The model under review builds one solid part; all positions refer to its coordinate system, in mm. A direction names the side the tool comes from. Round coordinates to 2 decimals unless told otherwise and drop trailing zeros. Order: outer loops, then holes, each group sorted by start corner. A loop starts at its lowest first (then second) coordinate and runs counter-clockwise, first axis right, second up. Notation, with made-up numbers: (-14, -34.5) - (6, -34.5) arc R5 ccw to (6, -28.5) - close; hole circle Ø9 at (29.25, -3.75). An arc over 180 degrees is marked (long way). One line per question, with ' | ' between items. Start each with the question number.
Item 1: Add section C-C on y = -4.25. State the section outline as (x, z) points.
Item 2: Draft analysis for pull direction Z (two halves, no side actions). For faces 3 (the face through (6.37, -0.94, 44.74)), 4 (the face through (4, -11, 0)), 5 (the face through (2.711, 9.938, 73.95)), state which applies: +Z half, -Z half, draft (parallel to the pull), parting line (faces both ways), or undercut.
Item 3: Insertion check: pin 1 Ø5 at (y, z) = (-0.01, 116.94) entering from -X; pin 2 Ø1.1 at (x, y) = (6, 0) entering from -Z; pin 3 Ø10 at (y, z) = (-6.5, 98) entering from -X. Each pin has a flat end and moves straight along its axis. Give the tip position at first contact, or say it passes through.
Item 4: For L1, parallel to Y at x = 2.5, z = 43.5; L2, parallel to X at y = 6, z = 116.5; L3, parallel to Y at x = 4, z = 23, list the stretches that pass through material, from the lowest coordinate up. Write a range as [from, to].
Item 5: Add section A-A on x = 2.5. State the section outline as (y, z) points, and give its area (3 significant figures).
Item 6: Tool access review of faces 1 (the face through (2.682, -9.952, 73.95)), 2 (the face through (2.686, 11.336, 73.95)): name each direction out of +Z, -Z, +X, -X, +Y, -Y from which nothing blocks a thin tool from reaching the whole face with its end or side.
Item 7: Add section B-B on z = 49.5. State the section outline as (x, y) points.
from build123d import *

# Parameters (mm, degrees)
BOSS_EXTRUDE1_DEPTH = 150
CUT_EXTRUDE2_DEPTH  = 151.642968673
SKETCH4_R           = 1.5
CUT_EXTRUDE3_DEPTH  = 151.642968673


with BuildPart() as part:
    # Sketch1 → Boss-Extrude1 (new body)
    with BuildSketch(Plane.XY):
        with BuildLine():
            Line((5.164341455, -10.750486483), (5.541822139, -10.750486483))
            ThreePointArc((5.541822139, -10.750486483), (5.628611698, -10.711655392), (5.6642, -10.623486496))
            Line((5.6642, -10.623486496), (5.6642, 10.623486496))
            ThreePointArc((5.6642, 10.623486496), (5.627002565, 10.713289048), (5.537200013, 10.750486483))
            Line((5.537200013, 10.750486483), (5.164341455, 10.750486483))
            ThreePointArc((5.164341455, 10.750486483), (5.123513594, 10.743744895), (5.087020295, 10.724235863))
            ThreePointArc((5.087020295, 10.724235863), (2.674694689, 9.938287609), (0.304054167, 10.842219578))
            Line((0.304054167, 10.842219578), (1.208194452, 11.907179363))
            ThreePointArc((1.208194452, 11.907179363), (2.709144677, 11.334862777), (4.236487447, 11.83247901))
            ThreePointArc((4.236487447, 11.83247901), (4.67440708, 12.066587417), (5.164341455, 12.147486483))
            Line((5.164341455, 12.147486483), (5.537200013, 12.147486483))
            ThreePointArc((5.537200013, 12.147486483), (6.614830738, 11.701117221), (7.0612, 10.623486496))
            Line((7.0612, 10.623486496), (7.0612, -10.623486496))
            ThreePointArc((7.0612, -10.623486496), (6.614830738, -11.701117221), (5.537200013, -12.147486483))
            ThreePointArc((5.537200013, -12.147486483), (5.350770734, -12.150925507), (5.164341455, -12.147486483))
            ThreePointArc((5.164341455, -12.147486483), (4.67440708, -12.066587417), (4.236487447, -11.83247901))
            ThreePointArc((4.236487447, -11.83247901), (2.709144677, -11.334862777), (1.208194452, -11.907179363))
            Line((1.208194452, -11.907179363), (0.304054167, -10.842219578))
            ThreePointArc((0.304054167, -10.842219578), (2.718249509, -9.951365406), (5.164341455, -10.750486483))
        make_face()
    extrude(amount=BOSS_EXTRUDE1_DEPTH)

    # Sketch2 → Cut-Extrude2 (cut, through all)
    with BuildSketch(Plane(origin=(7.0612, 0, 0), x_dir=(0, 0, -1), z_dir=(1, 0, 0))):
        with BuildLine():
            Line((0.119534124, 8.556064117), (0.119534124, -8.622507572))
            Line((0.119534124, -8.622507572), (-5.739792333, -7.254437811))
            ThreePointArc((-5.739792333, -7.254437811), (-6.226240725, -6.563404626), (-5.595417274, -6.001069606))
            Line((-5.595417274, -6.001069606), (-5.595417274, 5.934626152))
            ThreePointArc((-5.595417274, 5.934626152), (-6.226240725, 6.496961172), (-5.739792333, 7.187994357))
            Line((-5.739792333, 7.187994357), (0.119534124, 8.556064117))
        make_face()
    extrude(amount=-CUT_EXTRUDE2_DEPTH, mode=Mode.SUBTRACT)

    # Sketch4 → Cut-Extrude3 (cut, through all)
    with BuildSketch(Plane(origin=(7.0612, 0, 0), x_dir=(0, 0, -1), z_dir=(1, 0, 0))):
        with Locations((-116.937524646, -0.007606355)):
            Circle(SKETCH4_R)
        with Locations((-43.552387309, -0.024489344)):
            Circle(SKETCH4_R)
        with BuildLine():
            Line((-33.064580696, 1.474128733), (-33.064580696, -1.525871267))
            ThreePointArc((-33.064580696, -1.525871267), (-34.564580696, -3.025871267), (-36.064580696, -1.525871267))
            Line((-36.064580696, -1.525871267), (-36.064580696, 1.474128733))
            ThreePointArc((-36.064580696, 1.474128733), (-34.564580696, 2.974128733), (-33.064580696, 1.474128733))
        make_face()
        with BuildLine():
            Line((-128.12384742, 1.494967211), (-124.507385363, 1.494135207))
            ThreePointArc((-124.507385363, 1.494135207), (-123.007730493, -0.006209843), (-124.508075543, -1.505864713))
            Line((-124.508075543, -1.505864713), (-128.1245376, -1.50503271))
            ThreePointArc((-128.1245376, -1.50503271), (-129.62419247, -0.00468766), (-128.12384742, 1.494967211))
        make_face()
    extrude(amount=-CUT_EXTRUDE3_DEPTH, mode=Mode.SUBTRACT)


solid = part.part
Determined:
1) outline: (5.66, 5.6) - (7.06, 5.6) - (7.06, 150) - (5.66, 150) - close
2) face 3: undercut | face 4: -Z half | face 5: draft
3) pin 1: x = 5.66 | pin 2: z = 5.6 | pin 3: x = 0.3
4) L1: [-11.35, -9.96], [9.95, 11.35] | L2: [5.66, 7.06] | L3: [-11.67, -10.14], [10.14, 11.67]
5) outline: (-11.35, 0) - (-9.96, 0) - (-9.96, 150) - (-11.35, 150) - close; (9.95, 0) - (11.35, 0) - (11.35, 150) - (9.95, 150) - close | area: 419 mm2
6) face 1: +Z, -Z | face 2: +Z, -Z, +Y
7) outline: (0.3, -10.84) - (1.21, -11.91) arc R2.41 cw to (4.24, -11.83) arc R1.52 ccw to (5.16, -12.15) arc R5.05 ccw to (5.54, -12.15) arc R1.52 ccw to (7.06, -10.62) - (7.06, 10.62) arc R1.52 ccw to (5.54, 12.15) - (5.16, 12.15) arc R1.52 ccw to (4.24, 11.83) arc R2.41 cw to (1.21, 11.91) - (0.3, 10.84) arc R3.81 ccw to (5.09, 10.72) arc R0.13 cw to (5.16, 10.75) - (5.54, 10.75) arc R0.13 cw to (5.66, 10.62) - (5.66, -10.62) arc R0.13 cw to (5.54, -10.75) - (5.16, -10.75) arc R3.92 ccw to start
